Part model, mm, in its own coordinate system. A direction names the side the tool comes from. Round coordinates to 2 decimals unless told otherwise and drop trailing zeros. Loops run counter-clockwise (first coordinate to the right, second up) from the corner with the lowest first, then second, coordinate; pieces in that order, holes last. Notation, with made-up numbers: (16, 43.5) - (67, 43.5) arc R18 cw to (67, 74.5) - close; hole circle Ø4 at (62, 41). An arc over 180 degrees is marked (long way). Put each result on its own line as item: value.
from build123d import *

# Parameters (mm, degrees)
EXTRUDE_2_DEPTH        = 2.25
SKETCH_1_5_W           = 2
SKETCH_1_5_H           = 2
EXTRUDE_3_DEPTH        = 1
EXTRUDE_4_DEPTH        = 0.9
EXTRUDE_5_DEPTH        = 2.9
FILLET_1_R             = 1.2
FILLET_1_OF_MIRROR_2_R = 1.2


with BuildPart() as part:
    # 草图1 → 凸台-拉伸2 (new, symmetric)
    with BuildSketch(Plane(origin=(0, 0, 0), x_dir=(1, 0, 0), z_dir=(0, 1, 0))):
        with BuildLine():
            Line((-18.5, -1.5), (18.5, -1.5))
            ThreePointArc((18.5, -1.5), (19.207106781, -1.792893219), (19.5, -2.5))
            Line((19.5, -2.5), (19.5, -12.3))
            Line((19.5, -12.3), (21, -12.3))
            Line((21, -12.3), (21, -2.5))
            ThreePointArc((21, -2.5), (20.267766953, -0.732233047), (18.5, 0))
            Line((18.5, 0), (-18.5, 0))
            ThreePointArc((-18.5, 0), (-20.267766953, -0.732233047), (-21, -2.5))
            Line((-21, -2.5), (-21, -12.3))
            Line((-21, -12.3), (-19.5, -12.3))
            Line((-19.5, -12.3), (-19.5, -2.5))
            ThreePointArc((-19.5, -2.5), (-19.207106781, -1.792893219), (-18.5, -1.5))
        make_face()
    extrude(amount=EXTRUDE_2_DEPTH, both=True)

    # 草图1<5> → 凸台-拉伸3 (add, symmetric)
    with BuildSketch(Plane(origin=(0, 0, 0), x_dir=(1, 0, 0), z_dir=(0, 1, 0))):
        with Locations((0, -2.5)):
            Rectangle(SKETCH_1_5_W, SKETCH_1_5_H)
    extrude(amount=EXTRUDE_3_DEPTH, both=True)

    # 草图1<6> → 凸台-拉伸4 (add, symmetric)
    with BuildSketch(Plane(origin=(0, 0, 0), x_dir=(1, 0, 0), z_dir=(0, 1, 0))):
        Polygon((9.278174593, 7.778174593), (1.5, 0), (4.045584412, 0), (10.550966799, 6.505382387), align=None)
        Polygon((-4.045584412, 0), (-1.5, 0), (-9.278174593, 7.778174593), (-10.550966799, 6.505382387), align=None)
    extrude(amount=EXTRUDE_4_DEPTH, both=True)

    # 草图2 → 凸台-拉伸5 (add)
    with BuildSketch(Plane.ZY.offset(-19.5)):
        with BuildLine():
            Line((19.3, 4.478921871), (14.3, 4.478921871))
            ThreePointArc((14.3, 4.478921871), (12.885786438, 3.893135433), (12.3, 2.478921871))
            Line((12.3, 2.478921871), (12.3, -2.521078129))
            ThreePointArc((12.3, -2.521078129), (12.885786438, -3.935291691), (14.3, -4.521078129))
            Line((14.3, -4.521078129), (19.3, -4.521078129))
            ThreePointArc((19.3, -4.521078129), (20.714213562, -3.935291691), (21.3, -2.521078129))
            Line((21.3, -2.521078129), (21.3, 2.478921871))
            ThreePointArc((21.3, 2.478921871), (20.714213562, 3.893135433), (19.3, 4.478921871))
        make_face()
    extrude_5 = extrude(amount=-EXTRUDE_5_DEPTH)

    # 圆角1
    fillet_1_edges = [part.edges().sort_by_distance(p)[0] for p in [
        (22.4, 3.893135433, 12.885786438),
        (22.4, 4.478921871, 16.8),
        (22.4, 3.893135433, 20.714213562),
        (22.4, -0.021078129, 21.3),
        (22.4, -3.935291691, 20.714213562),
        (22.4, -4.521078129, 16.8),
        (22.4, -3.935291691, 12.885786438),
        (22.4, -0.021078129, 12.3),
    ]]
    fillet(fillet_1_edges, radius=FILLET_1_R)

    # 镜向2: 凸台-拉伸5 across plane
    add(extrude_5.mirror(Plane(origin=(0, 0, 0), x_dir=(0, 0, 1), z_dir=(1, 0, 0))))

    # 圆角1 of 镜向2
    fillet_1_of_mirror_2_edges = [part.edges().sort_by_distance(p)[0] for p in [
        (-22.4, 3.893135433, 12.885786438),
        (-22.4, 4.478921871, 16.8),
        (-22.4, 3.893135433, 20.714213562),
        (-22.4, -0.021078129, 21.3),
        (-22.4, -3.935291691, 20.714213562),
        (-22.4, -4.521078129, 16.8),
        (-22.4, -3.935291691, 12.885786438),
        (-22.4, -0.021078129, 12.3),
    ]]
    fillet(fillet_1_of_mirror_2_edges, radius=FILLET_1_OF_MIRROR_2_R)


solid = part.part
1. Probe line 1 along X through (y, z) = (3.25, 18.5); line 2 along X through (y, z) = (1.75, 12); line 3 along Z through (x, y) = (-3, 0.5). List the from-to ranges inside material, lowest first. Write a range as [from, to].
A:
line 1: x = [-22.4, -19.5], [19.5, 22.4]
line 2: x = [-21, -19.5], [19.5, 21]
line 3: z = [-1.5, 1.5]
2. Two-plate mould, pull along X, no slides. Class faces 1 (the flat face through (20, 4.479, 17)), 2 (the flat face through (-22.4, 0, 17)), 3 (the flat face through (1, 0, 3)), 4 (the cylindrical face through (22.039, 4.137, 16.765)): pulls with the +X half, pulls with the -X half, needs draft (parallel to the pull), parting line crosses it, or undercut.
A:
face 1: needs draft
face 2: pulls with the -X half
face 3: undercut
face 4: pulls with the +X half
3. Band-saw the part on D-D (z = -3.25). List the corners of the cut face in (x, y).
A:
outline: (-7.3, -0.9) - (-4.75, -0.9) - (-4.75, 0.9) - (-7.3, 0.9) - close; (4.75, -0.9) - (7.3, -0.9) - (7.3, 0.9) - (4.75, 0.9) - close
4. Band-saw the part on C-C (y = -1.75). List the corners of the cut face in (x, z), plus the area to 3 significant figures.
A:
outline: (-22.4, 13.5) arc R1.2 ccw to (-21.2, 12.3) - (-21, 12.3) - (-21, 2.5) arc R2.5 ccw to (-18.5, 0) - (18.5, 0) arc R2.5 ccw to (21, 2.5) - (21, 12.3) - (21.2, 12.3) arc R1.2 ccw to (22.4, 13.5) - (22.4, 20.1) arc R1.2 ccw to (21.2, 21.3) - (19.5, 21.3) - (19.5, 2.5) arc R1 cw to (18.5, 1.5) - (-18.5, 1.5) arc R1 cw to (-19.5, 2.5) - (-19.5, 21.3) - (-21.2, 21.3) arc R1.2 ccw to (-22.4, 20.1) - close
area: 144 mm²
5. Pin check, flat tips, straight feed: P1, Ø2.5, axis at x = -6.5, z = -5, coming from the +Y side; P2, Ø1.3, axis at y = -1, z = 6, coming from the -X side; P3, Ø1.6, axis at x = 0.5, z = 3, coming from the +Y side. Stop position of each tip, or through.
A:
P1: stops at y = 0.9
P2: stops at x = -21
P3: stops at y = 1
6. Tool access for faces 5 (the flat face through (7.253, -0.013, -3.207)), 6 (the cylindrical face through (-19.215, 0.031, 1.801)), 7 (the cylindrical face through (-22.039, -0.056, 12.642)), 8 (the flat face through (6, 0.9, -3)): list every direction of +Z, -Z, +X, -X, +Y, -Y with a clear straight run to the whole face (end or side of a thin tool).
A:
face 5: +X, +Y, -Y
face 6: +Z, +Y, -Y
face 7: -Z, -X, +Y, -Y
face 8: -Z, +X, -X, +Y
7. Band-saw the part on B-B (x = -6). List the corners of the cut face in (y, z).
A:
outline: (-2.25, 0) - (2.25, 0) - (2.25, 1.5) - (-2.25, 1.5) - close; (-0.9, -4.5) - (0.9, -4.5) - (0.9, -1.95) - (-0.9, -1.95) - close
8. Band-saw the part on A-A (z = 15.5). List the corners of the cut face in (x, y).
A:
outline: (-22.4, -3.32) arc R1.2 ccw to (-21.2, -4.52) - (-19.5, -4.52) - (-19.5, 4.48) - (-21.2, 4.48) arc R1.2 ccw to (-22.4, 3.28) - close; (19.5, -4.52) - (21.2, -4.52) arc R1.2 ccw to (22.4, -3.32) - (22.4, 3.28) arc R1.2 ccw to (21.2, 4.48) - (19.5, 4.48) - close
